Can you work these out from the model? Positions are in its coordinate system, mm. A direction names the side the tool comes from. Round coordinates to 2 decimals unless told otherwise and drop trailing zeros. Write each loop counter-clockwise with the first axis right and the second up, starting at its lowest first coordinate (ties: lowest second). Pieces come first, ordered by that corner, then holes. Notation, with made-up numbers: M 86,-10 L 136,-10 A28 cw 136,14 Z; hole C -8,85 d8. An arc over 180 degrees is marked long. Answer in a Markdown table with one row per item. Add a question column.
(1) Suppose I cut it at A-A, the plane x = -15. Write out the boundary of the cut face in (y, z).
(2) I'm going to push flat-ended pins straight in: pin 1 (4 mm diameter, centred on x = -14.5, y = 12.5, fed in from -Z); pin 2 (7.5 mm diameter, centred on y = 17, z = -9.5, fed in from -X); pin 3 (8 mm diameter, centred on x = -4.5, y = 52, fed in from -Z). Where does each tip first touch, or does it pass through?
(3) Suppose I cut it at B-B, the plane z = 17.5. Write out the boundary of the cut face in (x, y), then the cut area to 3 significant figures.
(4) If I drill on probe 1 along X at (y, z) = (43, 28); probe 2 along X at (y, z) = (29, -10.5); probe 3 along Y at (x, z) = (36, 34.5), over which ranges is the centre line in solid material (lowest first)?
(5) Suppose I cut it at D-D, the plane y = 33. Write out the boundary of the cut face in (x, z), then the cut area to 3 significant figures.
(6) Suppose I cut it at C-C, the plane y = 42.5. Write out the boundary of the cut face in (x, z), then the cut area to 3 significant figures.
(7) For faces 1 (the face through (-5, 19, 28)), 2 (the face through (20, 31, -12)), 3 (the face through (-20, 31, -12)), which set-ups out of +Z, -Z, +X, -X, +Y, -Y let a thin tool reach every point of the face, with its end or its side?
from build123d import *

# Parameters (mm, degrees)
CROQUIS2_W                   = 100
CROQUIS2_H                   = 100
CROQUIS2_W_2                 = 40
CROQUIS2_H_2                 = 40
SALIENTE_EXTRUIR1_DEPTH      = 2
CROQUIS2_2_W                 = 40
CROQUIS2_2_H                 = 40
SALIENTE_EXTRUIR2_DEPTH      = 60
SALIENTE_EXTRUIR3_DEPTH      = 5
SALIENTE_EXTRUIR3_DEPTH_BACK = 5
SALIENTE_EXTRUIR4_DEPTH      = 5
SALIENTE_EXTRUIR4_DEPTH_BACK = 5


with BuildPart() as part:
    # Croquis2 → Saliente-Extruir1 (new body)
    with BuildSketch(Plane(origin=(0, 0, 0), x_dir=(1, 0, 0), z_dir=(0, 1, 0))):
        Rectangle(CROQUIS2_W, CROQUIS2_H)
        Rectangle(CROQUIS2_W_2, CROQUIS2_H_2, mode=Mode.SUBTRACT)
    extrude(amount=SALIENTE_EXTRUIR1_DEPTH)

    # Croquis2<2> → Saliente-Extruir2 (add)
    with BuildSketch(Plane(origin=(0, 0, 0), x_dir=(1, 0, 0), z_dir=(0, 1, 0))):
        Rectangle(CROQUIS2_2_W, CROQUIS2_2_H)
    extrude(amount=SALIENTE_EXTRUIR2_DEPTH)

    # Croquis4 → Saliente-Extruir3 (add, two sides: drawn at the far end of the back side and taken through both)
    with BuildSketch(Plane(origin=(0, 0, 0), x_dir=(0, 0, -1), z_dir=(1, 0, 0)).offset(-SALIENTE_EXTRUIR3_DEPTH_BACK)):
        Polygon((20, 60), (50, 2), (20, 2), align=None)
        Polygon((-20, 2), (-50, 2), (-20, 60), align=None)
    extrude(amount=SALIENTE_EXTRUIR3_DEPTH + SALIENTE_EXTRUIR3_DEPTH_BACK)

    # Croquis5 → Saliente-Extruir4 (add, two sides: drawn at the far end of the back side and taken through both)
    with BuildSketch(Plane.XY.offset(-SALIENTE_EXTRUIR4_DEPTH_BACK)):
        Polygon((20, 60), (50, 2), (20, 2), align=None)
        Polygon((-20, 60), (-50, 2), (-20, 2), align=None)
    extrude(amount=SALIENTE_EXTRUIR4_DEPTH + SALIENTE_EXTRUIR4_DEPTH_BACK)


solid = part.part
Calculated:
| question | item | result |
|---|---|---|
| 1 | outline | M 0,-50 L 2,-50 L 2,-20 L 60,-20 L 60,20 L 2,20 L 2,50 L 0,50 Z |
| 2 | pin 1 | z = -20 |
| 2 | pin 2 | x = -20 |
| 2 | pin 3 | z = -26.21 |
| 3 | outline | M -50,0 L 50,0 L 50,2 L 20,2 L 20,60 L -20,60 L -20,2 L -50,2 Z |
| 3 | area | 2,520 mm² |
| 4 | probe 1 | -5 to 5 |
| 4 | probe 2 | -20 to 20 |
| 4 | probe 3 | 0 to 2 |
| 5 | outline | M -33.97,-5 L -20,-5 L -20,-20 L -5,-20 L -5,-33.97 L 5,-33.97 L 5,-20 L 20,-20 L 20,-5 L 33.97,-5 L 33.97,5 L 20,5 L 20,20 L 5,20 L 5,33.97 L -5,33.97 L -5,20 L -20,20 L -20,5 L -33.97,5 Z |
| 5 | area | 2,160 mm² |
| 6 | outline | M -29.05,-5 L -20,-5 L -20,-20 L -5,-20 L -5,-29.05 L 5,-29.05 L 5,-20 L 20,-20 L 20,-5 L 29.05,-5 L 29.05,5 L 20,5 L 20,20 L 5,20 L 5,29.05 L -5,29.05 L -5,20 L -20,20 L -20,5 L -29.05,5 Z |
| 6 | area | 1,960 mm² |
| 7 | face 1 | +Z, -X, +Y |
| 7 | face 2 | -Z, +X, +Y |
| 7 | face 3 | -Z, -X, +Y |
